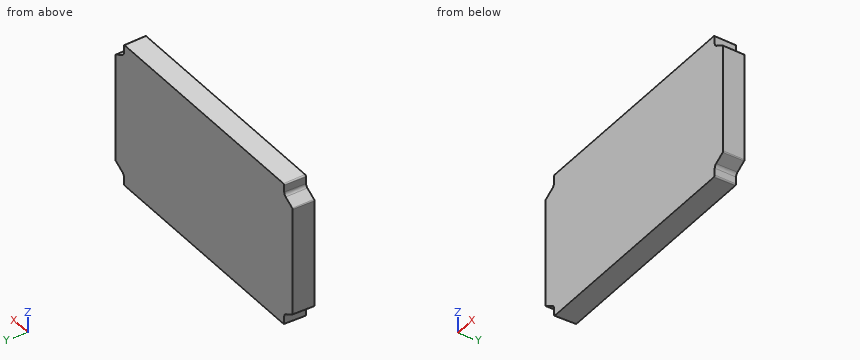
from build123d import *

# Parameters (mm, degrees)
BOSS_EXTRUDE1_DEPTH = 25
BOSS_EXTRUDE1_DRAFT = 1


with BuildPart() as part:
    # Sketch1 → Boss-Extrude1 (with draft: the straight prism first)
    with BuildSketch(Plane(origin=(0, -37.552068535, 0), x_dir=(1, 0, 0), z_dir=(0, 1, 0))):
        with BuildLine():
            ThreePointArc((150.559794425, 62.112181192), (150.39707932, 62.719442231), (149.952533386, 63.163988165))
            Line((149.952533386, 63.163988165), (138.703010202, 69.658903404))
            ThreePointArc((138.703010202, 69.658903404), (136.878930836, 71.482982769), (136.21127145, 73.97472152))
            Line((136.21127145, 73.97472152), (136.21127145, 82.121264476))
            ThreePointArc((136.21127145, 82.121264476), (135.855546169, 82.980061273), (134.996749372, 83.335786554))
            Line((134.996749372, 83.335786554), (-134.996749372, 83.335786554))
            ThreePointArc((-134.996749372, 83.335786554), (-135.855546169, 82.980061273), (-136.21127145, 82.121264476))
            Line((-136.21127145, 82.121264476), (-136.21127145, 73.97472152))
            ThreePointArc((-136.21127145, 73.97472152), (-136.878930836, 71.482982769), (-138.703010202, 69.658903404))
            Line((-138.703010202, 69.658903404), (-149.952533386, 63.163988165))
            ThreePointArc((-149.952533386, 63.163988165), (-150.39707932, 62.719442231), (-150.559794425, 62.112181192))
            Line((-150.559794425, 62.112181192), (-150.559794425, -62.112181192))
            ThreePointArc((-150.559794425, -62.112181192), (-150.39707932, -62.719442231), (-149.952533386, -63.163988165))
            Line((-149.952533386, -63.163988165), (-138.703010202, -69.658903404))
            ThreePointArc((-138.703010202, -69.658903404), (-136.878930836, -71.482982769), (-136.21127145, -73.97472152))
            Line((-136.21127145, -73.97472152), (-136.21127145, -82.121264476))
            ThreePointArc((-136.21127145, -82.121264476), (-135.855546169, -82.980061273), (-134.996749372, -83.335786554))
            Line((-134.996749372, -83.335786554), (134.996749372, -83.335786554))
            ThreePointArc((134.996749372, -83.335786554), (135.855546169, -82.980061273), (136.21127145, -82.121264476))
            Line((136.21127145, -82.121264476), (136.21127145, -73.97472152))
            ThreePointArc((136.21127145, -73.97472152), (136.878930836, -71.482982769), (138.703010202, -69.658903404))
            Line((138.703010202, -69.658903404), (149.952533386, -63.163988165))
            ThreePointArc((149.952533386, -63.163988165), (150.39707932, -62.719442231), (150.559794425, -62.112181192))
            Line((150.559794425, -62.112181192), (150.559794425, 62.112181192))
        make_face()
    extrude(amount=-BOSS_EXTRUDE1_DEPTH)
    # Boss-Extrude1: the draft: its side faces are tilted about the plane it starts from
    boss_extrude1_sides = [part.faces().sort_by_distance(p)[0] for p in [
        (150.39707932, -50.052068535, -62.719442231),
        (144.327771794, -50.052068535, -66.411445784),
        (136.878930836, -50.052068535, -71.482982769),
        (136.21127145, -50.052068535, -78.047992998),
        (135.855546169, -50.052068535, -82.980061273),
        (0, -50.052068535, -83.335786554),
        (-135.855546169, -50.052068535, -82.980061273),
        (-136.21127145, -50.052068535, -78.047992998),
        (-136.878930836, -50.052068535, -71.482982769),
        (-144.327771794, -50.052068535, -66.411445784),
        (-150.39707932, -50.052068535, -62.719442231),
        (-150.559794425, -50.052068535, 0),
        (-150.39707932, -50.052068535, 62.719442231),
        (-144.327771794, -50.052068535, 66.411445784),
        (-136.878930836, -50.052068535, 71.482982769),
        (-136.21127145, -50.052068535, 78.047992998),
        (-135.855546169, -50.052068535, 82.980061273),
        (0, -50.052068535, 83.335786554),
        (135.855546169, -50.052068535, 82.980061273),
        (136.21127145, -50.052068535, 78.047992998),
        (136.878930836, -50.052068535, 71.482982769),
        (144.327771794, -50.052068535, 66.411445784),
        (150.39707932, -50.052068535, 62.719442231),
        (150.559794425, -50.052068535, 0),
    ]]
    draft(boss_extrude1_sides, Plane(origin=(0, -37.552068535, 0), x_dir=(1, 0, 0), z_dir=(0, 1, 0)), BOSS_EXTRUDE1_DRAFT)


solid = part.part
The listing builds one solid part. Answer for the finished solid, in the listing's coordinates (mm). Give positions to 0.01 mm unless a question says otherwise; leave off trailing zeros. Write each loop counter-clockwise with the first axis right and the second up, starting at its lowest first coordinate (ties: lowest second). Pieces come first, ordered by that corner, then holes.
Item 1: Find the intervals of material crossed by line 1 along Z through (x, y) = (23, -40.75); line 2 along X through (y, z) = (-40.5, -29); line 3 along X through (y, z) = (-60.5, -29.5), in increasing order.
Item 2: Section B-B, the plane y = -42.75 is taken. Write down the section's boundary in (x, z).
Item 3: Flat-ended cylindrical pins translate along their axes: P1, Ø10, axis at x = 9.5, y = -55, coming from the -Z side; P2, Ø10, axis at x = 86.5, y = -49.5, coming from the +Z side; P3, Ø5, axis at y = -47, z = 43, coming from the +X side. Find the tip coordinate at first contact, or state that the pin passes through.
Item 4: Section A-A, the plane y = -59.75 is taken. Write down the section's boundary in (x, z).
Completed:
1. line 1: z = -83.39 to 83.39
1. line 2: x = -150.61 to 150.61
1. line 3: x = -150.96 to 150.96
2. outline: (-150.65, -62.11) arc R1.31 ccw to (-150, -63.24) - (-138.75, -69.74) arc R4.89 cw to (-136.3, -73.97) - (-136.3, -82.12) arc R1.31 ccw to (-135, -83.43) - (135, -83.43) arc R1.31 ccw to (136.3, -82.12) - (136.3, -73.97) arc R4.89 cw to (138.75, -69.74) - (150, -63.24) arc R1.31 ccw to (150.65, -62.11) - (150.65, 62.11) arc R1.31 ccw to (150, 63.24) - (138.75, 69.74) arc R4.89 cw to (136.3, 73.97) - (136.3, 82.12) arc R1.31 ccw to (135, 83.43) - (-135, 83.43) arc R1.31 ccw to (-136.3, 82.12) - (-136.3, 73.97) arc R4.89 cw to (-138.75, 69.74) - (-150, 63.24) arc R1.31 ccw to (-150.65, 62.11) - close
3. P1: stops at z = -83.73
3. P2: stops at z = 83.63
3. P3: stops at x = 150.77
4. outline: (-150.95, -62.11) arc R1.6 ccw to (-150.15, -63.5) - (-138.9, -69.99) arc R4.6 cw to (-136.6, -73.97) - (-136.6, -82.12) arc R1.6 ccw to (-135, -83.72) - (135, -83.72) arc R1.6 ccw to (136.6, -82.12) - (136.6, -73.97) arc R4.6 cw to (138.9, -69.99) - (150.15, -63.5) arc R1.6 ccw to (150.95, -62.11) - (150.95, 62.11) arc R1.6 ccw to (150.15, 63.5) - (138.9, 69.99) arc R4.6 cw to (136.6, 73.97) - (136.6, 82.12) arc R1.6 ccw to (135, 83.72) - (-135, 83.72) arc R1.6 ccw to (-136.6, 82.12) - (-136.6, 73.97) arc R4.6 cw to (-138.9, 69.99) - (-150.15, 63.5) arc R1.6 ccw to (-150.95, 62.11) - close
